Verification items for the finished model (mm, model axes). A direction names the side the tool comes from. Round coordinates to 2 decimals unless told otherwise and drop trailing zeros. Order: outer loops, then holes, each group sorted by start corner. A loop starts at its lowest first (then second) coordinate and runs counter-clockwise, first axis right, second up. Notation, with made-up numbers: M 8.5,85 L 34.5,85 A23 cw 34.5,95 Z; hole C 2.25,74 d4. An arc over 180 degrees is marked long. Answer as a JSON object with one key per item and string values. Group by question number.
```python
from build123d import *

# Parameters (mm, degrees)
EXTRUDE_1_DEPTH     = 350
CUT_EXTRUDE_1_DEPTH = 16


with BuildPart() as part:
    # Эскиз1 → Бобышка-Вытянуть1 (new body)
    with BuildSketch(Plane(origin=(0, 0, 0), x_dir=(0, 0, -1), z_dir=(1, 0, 0))):
        Polygon((0, 0), (0, 15), (1.5, 15), (1.5, 1.5), (15, 1.5), (15, 0), align=None)
    extrude(amount=EXTRUDE_1_DEPTH)

    # Эскиз2 → Вырез-Вытянуть1 (cut, through all)
    with BuildSketch(Plane.XY):
        Polygon((0, 0), (21.729873861, 21.729873861), (0, 21.729873861), align=None)
    cut_extrude_1 = extrude(amount=-CUT_EXTRUDE_1_DEPTH, mode=Mode.SUBTRACT)

    # Зеркальное отражение1: Вырез-Вытянуть1 across plane
    add(cut_extrude_1.mirror(Plane.ZY.offset(-175)), mode=Mode.SUBTRACT)


solid = part.part
```
Q1. Cross-section at A-A, the plane x = 200.5. Record the cut outline in (y, z).
Q2. Cross-section at B-B, the plane z = -7.5. Record the cut outline in (x, y).
Q3. Tool access check on faces 1 (the face through (173, 1.5, -8)), 2 (the face through (4, 4, -1)). Record the directions out of +Z, -Z, +X, -X, +Y, -Y that give a thin tool (end or side, any length) a straight path to the whole face; none if there is none.
Q4. Gauge pin test, flat ends, axial feed: pin 1 Ø4 at (x, z) = (102, -10) entering from +Y; pin 2 Ø3 at (y, z) = (7, -4.5) entering from +X; pin 3 Ø6 at (y, z) = (4, -3.5) entering from +X; pin 4 Ø4 at (x, y) = (114, 6.5) entering from -Z. Record the tip position at first contact, or that the pin passes through.
Q5. Thickness scan on line 1 (Z direction, x = 140, y = 13.25); line 2 (Y direction, x = 324, z = -4.75); line 3 (X direction, y = 10, z = -0.75). Record the ranges inside material, lowest first. Write a range as from..to.
Q6. Cross-section at C-C, the plane y = 4.5. Record the cut outline in (x, z), then the cut area to 4 significant figures.
Conclusion:
{
 "1": {"outline": "M 0,-15 L 1.5,-15 L 1.5,-1.5 L 15,-1.5 L 15,0 L 0,0 Z"},
 "2": {"outline": "M 0,0 L 350,0 L 348.5,1.5 L 1.5,1.5 Z"},
 "3": {"face 1": "-Z, +X, -X, +Y", "face 2": "+Z, -Z, -X, +Y"},
 "4": {"pin 1": "y = 1.5", "pin 2": "through", "pin 3": "x = 349", "pin 4": "z = -1.5"},
 "5": {"line 1": "-1.5..0", "line 2": "0..1.5", "line 3": "10..340"},
 "6": {"outline": "M 4.5,-1.5 L 345.5,-1.5 L 345.5,0 L 4.5,0 Z", "area": "511.5 mm2"}
}
